Geometry check sheet. Reference: the model listing, model coordinates, mm. Face numbers are marked on the shaded views. A direction names the side the tool comes from. Coordinates: 2 decimals unless noted, no trailing zeros. Write each loop counter-clockwise with the first axis right and the second up, starting at its lowest first coordinate (ties: lowest second). Pieces come first, ordered by that corner, then holes. Notation, with made-up numbers: (35, -17) -> (92, -17) arc R30 ccw to (92, 11) -> close; hole circle Ø11 at (-10.75, 87.25). An arc over 180 degrees is marked (long way). Answer in a Markdown table with one row per item. Add a question column.
1. Depth check by flat-ended pin: P1, Ø5.5, axis at y = 18.5, z = 1.5, coming from the -X side; P2, Ø18, axis at x = 11.5, y = 25.5, coming from the -Z side; P3, Ø3, axis at x = 9.5, y = 33.5, coming from the +Z side; P4, Ø8, axis at x = 11.5, y = 22, coming from the +Z side. Enter the tip coordinate at first touch or a pass-through.
2. Cross-section at A-A on z = 0. Record the cut outline in (x, y).
3. Cross-section at C-C on x = 5.5. Record the cut outline in (y, z), and give its area (3 significant figures).
4. Scan lines: L1, parallel to X at y = 15.5, z = -1.5; L2, parallel to Y at x = -5, z = -7.75; L3, parallel to X at y = 1.2, z = 0. Record each from-to range of solid material in increasing order. Write a range as from..to.
5. Cross-section at B-B on y = 7. Record the cut outline in (x, z), and give its area (3 significant figures).
6. Cross-section at D-D on y = 32.5. Record the cut outline in (x, z), and give its area (3 significant figures).
7. Set-up check for the marked faces 1, 2, 3, 4 and 5: record each of +Z, -Z, +X, -X, +Y, -Y from which the full face is reachable in a straight line by a thin tool's end or side.
8. Mould release check, pull along X, two halves, no side actions. Record for the marked faces 6, 7 and 8: pulls with the +X half, pulls with the -X half, needs draft (parallel to the pull), parting line crosses it, or undercut.
```python
from build123d import *

# Parameters (mm, degrees)
F2_DEPTH = 3.5
F1_R     = 11.798714
F1_R_2   = 6.798714
F3_DEPTH = 5
F4_SIZE  = 1.5


with BuildPart() as f2:
    # F0 (on Top) → F2 (new body, symmetric)
    with BuildSketch(Plane.XY):
        Polygon((5, 40), (0, 40), (0, 0), (16.2, 0), (16.2, 30.672841), (11.2, 30.672841), (11.2, 5.187817), (5, 5.187817), align=None)
    extrude(amount=F2_DEPTH, both=True)

    # F1 (on Front) → F3 (join)
    with BuildSketch(Plane.XZ):
        with Locations((-6.755837, 0)):
            Circle(F1_R)
        with Locations((-6.755837, 0)):
            Circle(F1_R_2, mode=Mode.SUBTRACT)
    extrude(amount=-F3_DEPTH)

    # F4
    f4_edges = [f2.edges().sort_by_distance(p)[0] for p in [
        (-18.554551, 0, 0),
        (-18.554551, 5, 0),
        (16.2, 0, 0),
        (10.3559, 0, -3.5),
        (10.3559, 0, 3.5),
        (16.2, 30.672841, 0),
        (0, 40, 0),
    ]]
    chamfer(f4_edges, length=F4_SIZE)


solid = f2.part
```
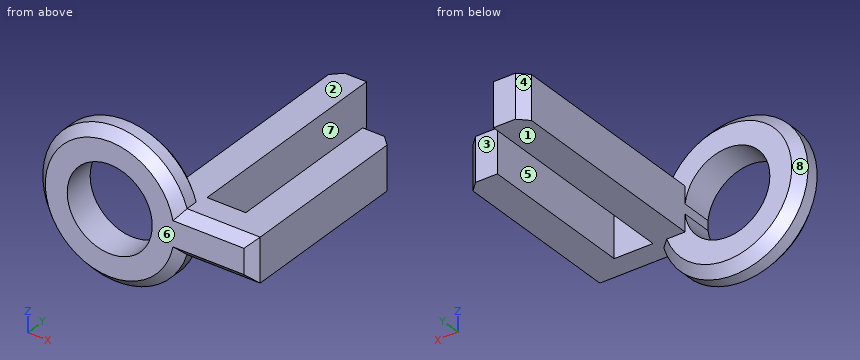
Results found:
| question | item | result |
|---|---|---|
| 1 | P1 | stops at x = 0 |
| 1 | P2 | stops at z = -3.5 |
| 1 | P3 | passes through |
| 1 | P4 | stops at z = 3.5 |
| 2 | outline | (-18.55, 1.5) -> (-17.05, 0) -> (-13.55, 0) -> (-13.55, 5) -> (-17.05, 5) -> (-18.55, 3.5) -> close; (0, 0) -> (14.7, 0) -> (16.2, 1.5) -> (16.2, 29.17) -> (14.7, 30.67) -> (11.2, 30.67) -> (11.2, 5.19) -> (5, 5.19) -> (5, 40) -> (1.5, 40) -> (0, 38.5) -> close |
| 3 | outline | (0, -2) -> (1.5, -3.5) -> (5.19, -3.5) -> (5.19, 3.5) -> (1.5, 3.5) -> (0, 2) -> close |
| 3 | area | 34.1 mm^2 |
| 4 | L1 | x = 0..5, 11.2..16.2 |
| 4 | L2 | y = 0..5 |
| 4 | L3 | x = -18.25..-13.55, 0..15.9 |
| 5 | outline | (0, -3.5) -> (5, -3.5) -> (5, 3.5) -> (0, 3.5) -> close; (11.2, -3.5) -> (16.2, -3.5) -> (16.2, 3.5) -> (11.2, 3.5) -> close |
| 5 | area | 70.0 mm^2 |
| 6 | outline | (0, -3.5) -> (5, -3.5) -> (5, 3.5) -> (0, 3.5) -> close |
| 6 | area | 35.0 mm^2 |
| 7 | face 1 | -Z, +X, +Y |
| 7 | face 2 | +Z, +X, +Y |
| 7 | face 3 | +Z, -Z, +X, +Y |
| 7 | face 4 | +Z, -Z, -X, +Y |
| 7 | face 5 | +Z, -Z, +Y |
| 8 | face 6 | needs draft |
| 8 | face 7 | undercut |
| 8 | face 8 | parting line crosses it |
